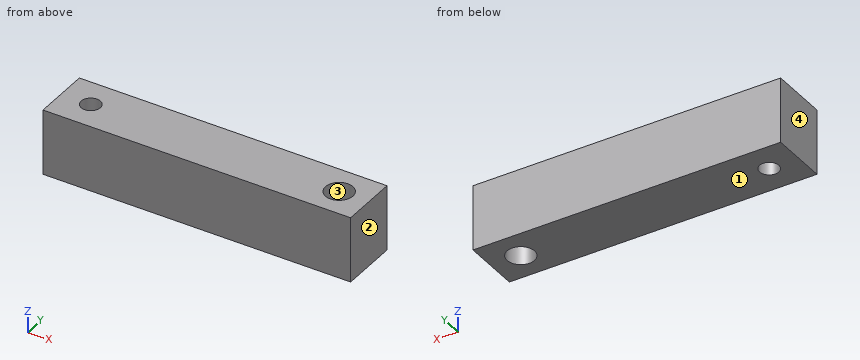
from build123d import *

# Parameters (mm, degrees)
BOSS_EXTRUDE1_START = 10
SKETCH1_W           = 80
SKETCH1_H           = 15
SKETCH1_R           = 3.57
SKETCH1_R_2         = 2.5
BOSS_EXTRUDE1_DEPTH = 17


with BuildPart() as part:
    # Sketch1 → Boss-Extrude1 (new body)
    with BuildSketch(Plane.XY.offset(BOSS_EXTRUDE1_START)):
        with Locations((0, 33.230865744)):
            Rectangle(SKETCH1_W, SKETCH1_H)
        with Locations((32.3, 33.230865744)):
            Circle(SKETCH1_R, mode=Mode.SUBTRACT)
        with Locations((-32.3, 33.230865744)):
            Circle(SKETCH1_R_2, mode=Mode.SUBTRACT)
    extrude(amount=BOSS_EXTRUDE1_DEPTH)


solid = part.part
For this review, take the finished solid that the model builds, in its own axes (mm). Face numbers are marked on the shaded views. Give positions to 0.01 mm unless a question says otherwise; leave off trailing zeros. Loops run counter-clockwise (first coordinate to the right, second up) from the corner with the lowest first, then second, coordinate; pieces in that order, holes last.
Item 1: Take a section at B-B, the plane y = 31.5. State the section outline as (x, z) points, and give its area (3 significant figures).
Item 2: Draft analysis for pull direction X (two halves, no side actions). For the marked faces 1, 2, 3 and 4, state which applies: +X half, -X half, draft (parallel to the pull), parting line (faces both ways), or undercut.
Item 3: Take a section at D-D, the plane z = 16.5. State the section outline as (x, y) points.
Item 4: Take a section at C-C, the plane x = -32.3. State the section outline as (y, z) points, and give its area (3 significant figures).
Item 5: Take a section at A-A, the plane x = 32.3. State the section outline as (y, z) points.
Item 6: For line 1 along X through (y, z) = (33.25, 16); line 2 along Y through (x, z) = (-32.3, 21.5); line 3 along Y through (x, z) = (32.3, 14.75), list the stretches that pass through material, from the lowest coordinate up.
Calculated:
1. outline: (-40, 10) - (-34.1, 10) - (-34.1, 27) - (-40, 27) - close; (-30.5, 10) - (29.18, 10) - (29.18, 27) - (-30.5, 27) - close; (35.42, 10) - (40, 10) - (40, 27) - (35.42, 27) - close
1. area: 1,190 mm2
2. face 1: draft
2. face 2: +X half
2. face 3: undercut
2. face 4: -X half
3. outline: (-40, 25.73) - (40, 25.73) - (40, 40.73) - (-40, 40.73) - close; hole circle Ø5 at (-32.3, 33.23); hole circle Ø7.14 at (32.3, 33.23)
4. outline: (25.73, 10) - (30.73, 10) - (30.73, 27) - (25.73, 27) - close; (35.73, 10) - (40.73, 10) - (40.73, 27) - (35.73, 27) - close
4. area: 170 mm2
5. outline: (25.73, 10) - (29.66, 10) - (29.66, 27) - (25.73, 27) - close; (36.8, 10) - (40.73, 10) - (40.73, 27) - (36.8, 27) - close
6. line 1: x = -40 to -34.8, -29.8 to 28.73, 35.87 to 40
6. line 2: y = 25.73 to 30.73, 35.73 to 40.73
6. line 3: y = 25.73 to 29.66, 36.8 to 40.73
